For this review, take the finished solid that the model builds, in its own axes (mm). A direction names the side the tool comes from. Give positions to 0.01 mm unless a question says otherwise; leave off trailing zeros. Write each loop counter-clockwise with the first axis right and the second up, starting at its lowest first coordinate (ties: lowest second). Pieces come first, ordered by that corner, then holes.
1) We need section A-A on x = 0. Give the boundary of the cut face in (y, z), and give its area (3 significant figures).
2) Draft analysis for pull direction Z (two halves, no side actions). For faces 1 (the face through (0.266, 2.699, 8.715)), 2 (the face through (5.2, 2, 6)), 3 (the face through (-28, 1, 0)), state which applies: pulls with the +Z half, pulls with the -Z half, needs draft (parallel to the pull), parting line crosses it, or undercut.
3) Wall thickness on line 1 along X through (y, z) = (0.85, 0); line 2 along X through (y, z) = (2.55, 1.25); line 3 along Z through (x, y) = (-4, 1.2): over which ranges is each line inside the solid? List them lowest first.
4) For P1, Ø0.6, axis at y = 2, z = 5.5, coming from the +X side; P2, Ø1.6, axis at y = 1, z = 6, coming from the -X side; P3, Ø3.5, axis at x = 19, z = 0, coming from the -Y side; P4, Ø2, axis at x = 19.5, z = 4, coming from the -Y side, all flat-tipped, find the tip position at first contact; note any pin that passes through.
5) We need section C-C on z = 0. Give the number of separate pieces and of enclosed holes in the cut face, and give its area (3 significant figures).
6) Machinability: for faces 4 (the face through (0, 0, -4)), 5 (the face through (-4, 2, -5.25)), which of the approach directions +Z, -Z, +X, -X, +Y, -Y give a long, thin tool a straight path to every point of the face, cutting with its end or side? Answer none if there is none.
7) We need section B-B on y = 0.8. Give the boundary of the cut face in (x, z).
from build123d import *

# Parameters (mm, degrees)
SKETCH1_R               = 2.25
SKETCH1_R_2             = 3.5
BOSS_EXTRUDE1_DEPTH     = 3
CUT_EXTRUDE1_DEPTH      = 30.563490998
CUT_EXTRUDE1_DEPTH_BACK = 30.563490998
SKETCH2_W               = 3
SKETCH2_H               = 2
FILLET1_R               = 1


with BuildPart() as part:
    # Sketch1 → Boss-Extrude1 (new body)
    with BuildSketch(Plane(origin=(0, 0, 0), x_dir=(1, 0, 0), z_dir=(0, 1, 0))):
        with BuildLine():
            Line((19, 9), (-19, 9))
            ThreePointArc((-19, 9), (-28, 0), (-19, -9))
            Line((-19, -9), (19, -9))
            ThreePointArc((19, -9), (28, 0), (19, 9))
        make_face()
        with Locations(Location((-19, 0, 0), (0, 0, 270))):
            Circle(SKETCH1_R, mode=Mode.SUBTRACT)
        with Locations(Location((19, 0, 0), (0, 0, 270))):
            Circle(SKETCH1_R, mode=Mode.SUBTRACT)
        with Locations(Location((0, -0.75, 0), (0, 0, 270))):
            Circle(SKETCH1_R_2, mode=Mode.SUBTRACT)
    extrude(amount=BOSS_EXTRUDE1_DEPTH)

    # Sketch2 → Cut-Extrude1 (cut, two sides: drawn at the far end of the back side and taken through both)
    with BuildSketch(Plane.XZ.offset(-CUT_EXTRUDE1_DEPTH_BACK)):
        with Locations((3.7, 5.75)):
            Rectangle(SKETCH2_W, SKETCH2_H)
        with Locations((-3.7, -4.25)):
            Rectangle(SKETCH2_W, SKETCH2_H)
    extrude(amount=CUT_EXTRUDE1_DEPTH + CUT_EXTRUDE1_DEPTH_BACK, mode=Mode.SUBTRACT)

    # Fillet1
    fillet1_edges = [part.edges().sort_by_distance(p)[0] for p in [
        (-19, 3, -2.25),
        (28, 3, 0),
        (19, 3, -2.25),
        (0, 3, -9),
        (0, 3, -2.75),
        (-28, 3, 0),
        (0, 3, 9),
    ]]
    fillet(fillet1_edges, radius=FILLET1_R)


solid = part.part
Results list:
1. outline: (0, -9) - (2, -9) arc R1 ccw to (3, -8) - (3, -3.75) arc R1 ccw to (2, -2.75) - (0, -2.75) - close; (0, 4.25) - (2, 4.25) arc R1 ccw to (3, 5.25) - (3, 8) arc R1 ccw to (2, 9) - (0, 9) - close
1. area: 32.1 mm2
2. face 1: pulls with the +Z half
2. face 2: undercut
2. face 3: parting line crosses it
3. line 1: x = -28 to -21.25, -16.75 to -3.42, 3.42 to 16.75, 21.25 to 28
3. line 2: x = -27.75 to -21.07, -16.93 to -3.63, 3.63 to 16.93, 21.07 to 27.75
3. line 3: z = -9 to -5.25, -3.25 to 9
4. P1: stops at x = 26.35
4. P2: stops at x = -26.35
4. P3: passes through
4. P4: stops at y = 0
5. separate pieces: 4
5. enclosed holes: 0
5. area: 119 mm2
6. face 4: +Z, -Z, +X, -X, -Y
6. face 5: +Y, -Y
7. outline: (-19, -9) - (19, -9) arc R9 ccw to (19, 9) - (-19, 9) arc R9 ccw to start; hole circle Ø4.5 at (-19, 0); hole (-5.2, -5.25) - (-2.2, -5.25) - (-2.2, -3.25) - (-5.2, -3.25) - close; hole circle Ø7 at (0, 0.75); hole (2.2, 4.75) - (5.2, 4.75) - (5.2, 6.75) - (2.2, 6.75) - close; hole circle Ø4.5 at (19, 0)
